Work out the finished part from the listing and answer in its coordinate system (mm). A direction names the side the tool comes from. Coordinates: 2 decimals unless noted, no trailing zeros. Loops run counter-clockwise (first coordinate to the right, second up) from the corner with the lowest first, then second, coordinate; pieces in that order, holes last. Notation, with made-up numbers: (-2.75, 80) -> (9.25, 80) arc R5 ccw to (9.25, 89) -> close; hole circle Ø9 at (0.25, -2.75). An arc over 180 degrees is marked (long way). Answer as CSV lines item,"result".
Autodesk Inventor part; units mm, degrees
ref_plane "Work Plane1" through (29, 0, 0) normal (0, -1, 0) x (1, 0, 0)
ref_plane "YZ Plane" through (0, 0, 0) normal (1, 0, 0) x (0, 1, 0)
ref_plane "XZ Plane" through (0, 0, 0) normal (0, 1, 0) x (-1, 0, 0)
sketch "Sketch1" plane through (0, 0, 0) normal (0, 0, 1) x (1, 0, 0)
  line L0 (0.0567, 0) -> (10, 0)
  line L1 (10, 0) -> (10, 1.5)
  line L2 (10, 1.5) -> (1, 1.5)
  line L3 (1, 1.5) -> (0.6932, 1.5)
  line L4 (0.6932, 1.5) -> (0, 1.5)
  line L5 (0, 1.5) -> (0, 2.85)
  line L6 (0, 2.85) -> (-1.65, 2.85)
  line L7 (-1.65, 2.85) -> (-1.65, 1.1547)
  line L8 (-1.65, 1.1547) -> (-0.61, 1.1547)
  line L9 (-0.61, 1.1547) -> (0.0567, 0)
  line L10 (-3.98, 0) -> (12.33, 0)
  line L11 (0, -0.57) -> (0, 3.42)
  line L12 (1, 1.5) -> (0, 1.5) construction
  dimension "d1" = 9
  dimension "d2" = 0.3068
  dimension "d3" = 1.65
  dimension "d4" = 1.04
  dimension "d5" = 60
  dimension "d6" = 3
  dimension "d7" = 3
  dimension "d8" = 2.3094
  dimension "d9" = 5.7
  dimension "d26" = 10
revolve "Body" add sketch "Sketch1" angle 360 about axis through (0.0567, 0, 0) along (1, 0, 0) contours L9 L11 L4 L3 L2 L1 L0 | L9 L8 L7 L6 L5 L11
sketch "Sketch2" plane through (-1.65, 0, 0) normal (-1, 0, 0) x (0, 0, 1)
  circle A0 centre (0, 0) radius 1.1547
  line L0 (0, -3.99) -> (0, 3.99)
  line L1 (-3.99, 0) -> (3.99, 0)
  line L2 (1.1547, 0) -> (0.5774, -1)
  line L3 (0.5774, -1) -> (-0.5774, -1)
  line L4 (-0.5774, -1) -> (-1.1547, 0)
  line L5 (-1.1547, 0) -> (-0.5774, 1)
  line L6 (-0.5774, 1) -> (0.5774, 1)
  line L7 (0.5774, 1) -> (1.1547, 0)
extrude "Slot" add sketch "Sketch2" against normal up to next contours L7 A0 | A0 L2 | L6 L0 A0 | A0 L0 L3 | L0 L6 A0 | A0 L3 L0 | L4 A0 | A0 L5
fillet "Fillet1" radius 1.45 1 edges at (-1.65, -2.85, 0)
thread "Thread"
chamfer "Chamfer1" distance 0.3067 distance2 0.3067 1 edges at (10, -1.5, 0) measured on face at (10, -0.6587, -0.1791)
ref_plane "Work Plane1" through (29, 0, 0) normal (0, -1, 0) x (1, 0, 0)
fillet "Fillet2" radius 0.1 1 edges at (0, -1.5, 0)
equation "\"d1\" = GEL"
equation "\"d3\" = KOH"
equation "\"d4\" = INTI"
equation "\"d6\" = GD"
equation "\"d7\" = BDM"
equation "\"d8\" = 1.1547 * SW"
equation "\"d9\" = KOD"
equation "\"d26\" = NLG"
equation "\"d30\" = R"
equation "\"d17\" = RR"
equation "\"d13\" = GEL"
equation "\"d15\" = -0.5 * SPD + 0.5 * GD"
equation "\"d16\" = GUL"
equation "\"GD\" = 3"
equation "\"NLG\" = 10"
equation "\"GEL\" = 9"
equation "\"KOD\" = 5.7"
equation "\"KOH\" = 1.65"
equation "\"INTI\" = 1.04"
equation "\"GAL\" = 0.30673"
equation "\"GUL\" = 0.30673"
equation "\"BDM\" = 3"
equation "\"SW\" = 2"
equation "\"RR\" = 1.45"
equation "\"SPD\" = 2.38655"
equation "\"R\" = 0.1"
equation "\"TOA\" = 30deg"
equation "\"GD1\" = 2.38655"
equation "\"THREADDIA\" = 3"
equation "\"PTC\" = 0.5"
equation "\"NND\" = 3"
equation "\"KOH1\" = 0.2"
equation "\"E0\" = 2.31"
properties part number "M3 x 10 - Socket Button Head (A2)" material "Steel, Alloy"
(1) A cutting plane is placed at A-A, the plane x = 4.75. Write down the section's boundary in (y, z), and give its area (3 significant figures).
Computed values:
outline,"circle Ø3 at (0, 0)"
area,"7.07 mm2"
(2) Which of the six approach directions +Z, -Z, +X, -X, +Y, -Y give full straight-line access (tool end or side, diameter ignored) to faces 1 (the face through (-1.09, -0.49, 0.87)), 2 (the face through (10, 0, 0))?
Computed values:
face 1,"-X"
face 2,"+Z, -Z, +X, +Y, -Y"
(3) Consider line 1 along Z through (x, y) = (2.25, 0.1); line 2 along X through (y, z) = (-0.3, -1.8). Determine where each line is inside the solid, lowest interval first.
Computed values:
line 1,"-1.5 to 1.5"
line 2,"-1.59 to 0"
(4) Flat-ended cylindrical pins translate along their axes: pin 1 Ø1.2 at (x, z) = (-1, -0.5) entering from -Y; pin 2 Ø0.6 at (x, z) = (-1.5, 0) entering from +Y; pin 3 Ø3 at (y, z) = (1.5, 1) entering from -X; pin 4 Ø1 at (x, y) = (8.5, 1.5) entering from -Z. Find the tip coordinate at first contact, or state that the pin passes through.
Computed values:
pin 1,"y = -2.82"
pin 2,"y = 2.45"
pin 3,"x = -1.65"
pin 4,"z = -1.12"
(5) For a pull along Z with two mould halves and no side action, classify faces 3 (the face through (4.83, -1.5, -0.07)), 4 (the face through (0, 0, -2)), 5 (the face through (-1.09, 0.49, -0.87)) as pulls with the +Z half, pulls with the -Z half, needs draft (parallel to the pull), parting line crosses it, or undercut.
Computed values:
face 3,"parting line crosses it"
face 4,"needs draft"
face 5,"undercut"
